```python
from build123d import *

# Parameters (mm, degrees)
SKETCH1_W           = 190
SKETCH1_H           = 275
BOSS_EXTRUDE1_DEPTH = 10
SKETCH2_W           = 125
SKETCH2_H           = 5
BOSS_EXTRUDE2_DEPTH = 5
SKETCH3_R           = 10
CUT_EXTRUDE1_DEPTH  = 16


with BuildPart() as part:
    # Sketch1 → Boss-Extrude1 (new body)
    with BuildSketch(Plane.XY):
        Rectangle(SKETCH1_W, SKETCH1_H)
    extrude(amount=BOSS_EXTRUDE1_DEPTH)

    # Sketch2 → Boss-Extrude2 (add)
    with BuildSketch(Plane(origin=(0, 137.5, 0), x_dir=(1, 0, 0), z_dir=(0, 1, 0))):
        with Locations((0, -5)):
            Rectangle(SKETCH2_W, SKETCH2_H)
    extrude(amount=BOSS_EXTRUDE2_DEPTH)

    # Sketch3 → Cut-Extrude1 (cut)
    with BuildSketch(Plane.XY.offset(10)):
        with Locations((0, -117.5)):
            Circle(SKETCH3_R)
        with Locations((-70, 107.5)):
            Circle(SKETCH3_R)
    extrude(amount=-CUT_EXTRUDE1_DEPTH, mode=Mode.SUBTRACT)


solid = part.part
```
Build history of the part. All positions in model axes, mm. Round coordinates to 2 decimals unless told otherwise and drop trailing zeros. Write each loop counter-clockwise with the first axis right and the second up, starting at its lowest first coordinate (ties: lowest second). Pieces come first, ordered by that corner, then holes. Notation, with made-up numbers: (86.5, -7) - (101.5, -7) arc R16 ccw to (101.5, 22) - close; hole circle Ø9 at (-34.5, -30.75). An arc over 180 degrees is marked (long way). Write each question's results on one line, items separated by ' | '. Start each with the question number.
Item 1: Mould opens along Y. For faces 1 (the face through (-77.37, 114.26, 5.07)), 2 (the face through (-1, -137.5, 5)), 3 (the face through (-1, 2, 0)) say: pulls with the +Y half, pulls with the -Y half, needs draft (parallel to the pull), parting line crosses it, or undercut.
Item 2: Saw through at C-C (x = -70). Write the cut outline in (y, z).
Item 3: Saw through at B-B (y = -117.5). Write the cut outline in (x, z), and give its area (3 significant figures).
Item 4: Saw through at A-A (z = 5.75). Write the cut outline in (x, y).
Item 5: Drop flat-ended pins along their axis: P1, Ø1.5, axis at y = 139.5, z = 5.5, coming from the +X side; P2, Ø1.5, axis at x = 54.5, z = 9, coming from the +Y side; P3, Ø2.5, axis at x = -14, y = 139, coming from the +Z side. Give the stop position or say it passes through.
Item 6: Wall check: L1, parallel to Y at x = 0, z = 5.75; L2, parallel to Y at x = -70, z = 4.75; L3, parallel to Y at x = 71, z = 5.25. Give the ranges that are in metal, low to high. Write a range as [from, to].
Results are:
1) face 1: undercut | face 2: pulls with the -Y half | face 3: needs draft
2) outline: (-137.5, 0) - (97.5, 0) - (97.5, 10) - (-137.5, 10) - close; (117.5, 0) - (137.5, 0) - (137.5, 10) - (117.5, 10) - close
3) outline: (-95, 0) - (-10, 0) - (-10, 10) - (-95, 10) - close; (10, 0) - (95, 0) - (95, 10) - (10, 10) - close | area: 1,700 mm²
4) outline: (-95, -137.5) - (95, -137.5) - (95, 137.5) - (62.5, 137.5) - (62.5, 142.5) - (-62.5, 142.5) - (-62.5, 137.5) - (-95, 137.5) - close; hole circle Ø20 at (-70, 107.5); hole circle Ø20 at (0, -117.5)
5) P1: stops at x = 62.5 | P2: stops at y = 137.5 | P3: stops at z = 7.5
6) L1: y = [-137.5, -127.5], [-107.5, 142.5] | L2: y = [-137.5, 97.5], [117.5, 137.5] | L3: y = [-137.5, 137.5]
